Work out the finished part from the listing and answer in its coordinate system (mm). Face numbers are marked on the shaded views. A direction names the side the tool comes from. Give positions to 0.01 mm unless a question says otherwise; leave off trailing zeros. Loops run counter-clockwise (first coordinate to the right, second up) from the corner with the lowest first, then second, coordinate; pieces in that order, holes last.
from build123d import *

# Parameters (mm, degrees)
PAD033_DEPTH                = 10
PAD032_DEPTH                = 10
BOX026_W                    = 12
BOX026_H                    = 10
BOX026_DEPTH                = 30
CYLINDER036_R               = 2.2
CYLINDER036_DEPTH           = 18
CYLINDER036_ROLL_ANGLE      = -90
ARRAY006_X_COUNT            = 2
ARRAY006_X_PITCH            = 49.2
ARRAY006_Z_COUNT            = 2
ARRAY006_Z_PITCH            = 10.3
PAD021_DEPTH                = 6
PAD020_DEPTH                = 10
BOX027_W                    = 12
BOX027_H                    = 10
BOX027_DEPTH                = 30
CYLINDER037_R               = 2.2
CYLINDER037_DEPTH           = 18
CYLINDER037_ROLL_ANGLE      = -90
ARRAY007_X_COUNT            = 2
ARRAY007_X_PITCH            = 49.2
ARRAY007_Z_COUNT            = 2
ARRAY007_Z_PITCH            = 10.3
PAD023_DEPTH                = 6
PAD022_DEPTH                = 10
BOX025_W                    = 16.3
BOX025_H                    = 10
BOX025_DEPTH                = 17
SKETCH018_R                 = 3
PAD018_DEPTH                = 4
SKETCH019_R                 = 3
PAD019_DEPTH                = 4
BOX024_W                    = 20
BOX024_H                    = 17
BOX024_DEPTH                = 10
FILLET007_R                 = 1
FILLET007_ROLL_ANGLE        = 90
FILLET008_1_R               = 2
FILLET008_2_R               = 1
BOX018_W                    = 16.3
BOX018_H                    = 10
BOX018_DEPTH                = 17
SKETCH010_R                 = 3
PAD010_DEPTH                = 4
SKETCH011_R                 = 3
PAD011_DEPTH                = 4
BOX016_W                    = 20
BOX016_H                    = 17
BOX016_DEPTH                = 10
FILLET005_R                 = 1
FILLET005_ROLL_ANGLE        = 90
FILLET006_1_R               = 2
FILLET006_2_R               = 1
PAD009_DEPTH                = 26.3
FUSION009003041_PITCH_ANGLE = 90


with BuildPart() as obj1:
    # Sketch033 → Pad033 (new body)
    with BuildSketch(Plane(origin=(-28, -127, 4), x_dir=(1, 0, 0), z_dir=(0, 0, 1))):
        Polygon((0, 0), (0, 6), (26, 6), (26, 0), (23, 0), (23, 3), (3, 3), (3, 0), align=None)
    extrude(amount=PAD033_DEPTH)


with BuildPart() as obj1_mirror:
    # Part__Mirroring009: instance of obj1
    add(obj1.part.mirror(Plane(origin=(0, 0, 0), x_dir=(1, 0, 0), z_dir=(0, 1, 0))))


with BuildPart() as obj1_mirror_1:
    # Part__Mirroring009 placement: moved
    add(obj1_mirror.part.moved(Location((0, -130, 0))))


with BuildPart() as obj2:
    # Sketch032 → Pad032 (new body)
    with BuildSketch(Plane(origin=(-28, -127, 4), x_dir=(1, 0, 0), z_dir=(0, 0, 1))):
        Polygon((0, 0), (0, 6), (26, 6), (26, 0), (23, 0), (23, 3), (3, 3), (3, 0), align=None)
    extrude(amount=PAD032_DEPTH)

    # Fusion009003040: union obj1_mirror
    add(obj1_mirror_1.part)


with BuildPart() as obj3:
    # Box026 → Box026 (new body)
    with BuildSketch(Plane(origin=(-29.5, -13, 0), x_dir=(1, 0, 0), z_dir=(0, 0, 1))):
        with Locations((6, 5)):
            Rectangle(BOX026_W, BOX026_H)
    extrude(amount=BOX026_DEPTH)


with BuildPart() as obj4:
    # Cylinder036 → Cylinder036 (new body)
    with BuildSketch(Plane.XY):
        Circle(CYLINDER036_R)
    extrude(amount=CYLINDER036_DEPTH)


with BuildPart() as obj4_1:
    # Cylinder036 roll: moved
    add(obj4.part.rotate(Axis((0, 0, 0), (1, 0, 0)), CYLINDER036_ROLL_ANGLE))


with BuildPart() as obj4_2:
    # Cylinder036 placement: moved
    add(obj4_1.part.moved(Location((150.075, 41, 13.5))))

    # Array006 X: obj4_2


with BuildPart() as obj4_3:
    add(obj4_2.part)
    with Locations(*[(i * ARRAY006_X_PITCH, 0, 0) for i in range(1, ARRAY006_X_COUNT)]):
        add(obj4_2.part)

    # Array006 Z: obj4_2


with BuildPart() as obj4_4:
    add(obj4_3.part)
    with Locations(*[(0, 0, -i * ARRAY006_Z_PITCH) for i in range(1, ARRAY006_Z_COUNT)]):
        add(obj4_3.part)


with BuildPart() as obj5:
    # Sketch021 → Pad021 (new body)
    with BuildSketch(Plane(origin=(10, 54.8, 0), x_dir=(1, 0, 0), z_dir=(0, -1, 0))):
        Polygon((0, 18.5), (0, 24.5), (50.5, 24.5), (50.5, 0), (40.5, 0), (40.5, 18.5), align=None)
    extrude(amount=PAD021_DEPTH)


with BuildPart() as obj6:
    # Sketch020 → Pad020 (new body)
    with BuildSketch(Plane.YZ):
        Polygon((14, 0), (0, 0), (0, 24.5), (54.8, 24.5), (54.8, 0), (48.8, 0), (48.8, 18.5), (14, 18.5), align=None)
    extrude(amount=PAD020_DEPTH)

    # Fusion009003025: union obj5
    add(obj5.part)


with BuildPart() as obj6_1:
    # Fusion009003025 placement: moved
    add(obj6.part.moved(Location((144.425, -3, 0))))

    # Cut017: cut obj4
    add(obj4_4.part, mode=Mode.SUBTRACT)


with BuildPart() as obj6_2:
    # Cut017 placement: moved
    add(obj6_1.part.moved(Location((-172.725, -4, 0))))

    # Cut018: cut obj3
    add(obj3.part, mode=Mode.SUBTRACT)


with BuildPart() as obj7:
    # Box027 → Box027 (new body)
    with BuildSketch(Plane(origin=(-29.5, -13, 0), x_dir=(1, 0, 0), z_dir=(0, 0, 1))):
        with Locations((6, 5)):
            Rectangle(BOX027_W, BOX027_H)
    extrude(amount=BOX027_DEPTH)


with BuildPart() as obj8:
    # Cylinder037 → Cylinder037 (new body)
    with BuildSketch(Plane.XY):
        Circle(CYLINDER037_R)
    extrude(amount=CYLINDER037_DEPTH)


with BuildPart() as obj8_1:
    # Cylinder037 roll: moved
    add(obj8.part.rotate(Axis((0, 0, 0), (1, 0, 0)), CYLINDER037_ROLL_ANGLE))


with BuildPart() as obj8_2:
    # Cylinder037 placement: moved
    add(obj8_1.part.moved(Location((150.075, 41, 13.5))))

    # Array007 X: obj8_2


with BuildPart() as obj8_3:
    add(obj8_2.part)
    with Locations(*[(i * ARRAY007_X_PITCH, 0, 0) for i in range(1, ARRAY007_X_COUNT)]):
        add(obj8_2.part)

    # Array007 Z: obj8_2


with BuildPart() as obj8_4:
    add(obj8_3.part)
    with Locations(*[(0, 0, -i * ARRAY007_Z_PITCH) for i in range(1, ARRAY007_Z_COUNT)]):
        add(obj8_3.part)


with BuildPart() as obj9:
    # Sketch023 → Pad023 (new body)
    with BuildSketch(Plane(origin=(10, 54.8, 0), x_dir=(1, 0, 0), z_dir=(0, -1, 0))):
        Polygon((0, 18.5), (0, 24.5), (50.5, 24.5), (50.5, 0), (40.5, 0), (40.5, 18.5), align=None)
    extrude(amount=PAD023_DEPTH)


with BuildPart() as obj10:
    # Sketch022 → Pad022 (new body)
    with BuildSketch(Plane.YZ):
        Polygon((14, 0), (0, 0), (0, 24.5), (54.8, 24.5), (54.8, 0), (48.8, 0), (48.8, 18.5), (14, 18.5), align=None)
    extrude(amount=PAD022_DEPTH)

    # Fusion009003026: union obj9
    add(obj9.part)


with BuildPart() as obj10_1:
    # Fusion009003026 placement: moved
    add(obj10.part.moved(Location((144.425, -3, 0))))

    # Cut019: cut obj8
    add(obj8_4.part, mode=Mode.SUBTRACT)


with BuildPart() as obj10_2:
    # Cut019 placement: moved
    add(obj10_1.part.moved(Location((-172.725, -4, 0))))

    # Cut020: cut obj7
    add(obj7.part, mode=Mode.SUBTRACT)


with BuildPart() as obj11:
    # Part__Mirroring: instance of obj10
    add(obj10_2.part.mirror(Plane(origin=(0, 0, 0), x_dir=(1, 0, 0), z_dir=(0, 1, 0))))


with BuildPart() as obj11_1:
    # Part__Mirroring placement: moved
    add(obj11.part.moved(Location((0, -130, 0))))


with BuildPart() as obj12:
    # Box025 → Box025 (new body)
    with BuildSketch(Plane(origin=(-26.3, -8, 0), x_dir=(1, 0, 0), z_dir=(0, 0, 1))):
        with Locations((8.15, 5)):
            Rectangle(BOX025_W, BOX025_H)
    extrude(amount=BOX025_DEPTH)


with BuildPart() as obj13:
    # Sketch018 → Pad018 (new body)
    with BuildSketch(Plane.XY):
        with BuildLine():
            Line((0, 17), (20, 17))
            ThreePointArc((20, 0), (28.500019, 8.5), (20, 17))
            Line((20, 0), (0, 0))
            Line((0, 0), (0, 17))
        make_face()
        with Locations((20.000019, 8.5)):
            Circle(SKETCH018_R, mode=Mode.SUBTRACT)
    extrude(amount=PAD018_DEPTH)


with BuildPart() as obj14:
    # Sketch019 → Pad019 (new body)
    with BuildSketch(Plane.XY.offset(14)):
        with BuildLine():
            Line((0, 17), (20, 17))
            ThreePointArc((20, 0), (28.500019, 8.5), (20, 17))
            Line((20, 0), (0, 0))
            Line((0, 0), (0, 17))
        make_face()
        with Locations((20.000019, 8.5)):
            Circle(SKETCH019_R, mode=Mode.SUBTRACT)
    extrude(amount=PAD019_DEPTH)


with BuildPart() as obj15:
    # Box024 → Box024 (new body)
    with BuildSketch(Plane(origin=(-16, 0, 4), x_dir=(1, 0, 0), z_dir=(0, 0, 1))):
        with Locations((10, 8.5)):
            Rectangle(BOX024_W, BOX024_H)
    extrude(amount=BOX024_DEPTH)

    # Fusion009003021: union obj13, obj14
    add(obj13.part)
    add(obj14.part)

    # Fillet007
    fillet007_edges = [obj15.edges().sort_by_distance(p)[0] for p in [
        (0, 8.5, 18),
        (-16, 0, 9),
        (-16, 17, 9),
        (0, 8.5, 0),
    ]]
    fillet(fillet007_edges, radius=FILLET007_R)


with BuildPart() as obj15_1:
    # Fillet007 roll: moved
    add(obj15.part.rotate(Axis((0, 0, 0), (1, 0, 0)), FILLET007_ROLL_ANGLE))


with BuildPart() as obj15_2:
    # Fillet007 placement: moved
    add(obj15_1.part.moved(Location((16, 15, 0))))

    # Fillet008 1
    fillet008_1_edges = [obj15_2.edges().sort_by_distance(p)[0] for p in [
        (16, 1, 8.5),
        (16, 11, 8.5),
    ]]
    fillet(fillet008_1_edges, radius=FILLET008_1_R)

    # Fillet008 2
    fillet008_2_edges = [obj15_2.edges().sort_by_distance(p)[0] for p in [
        (20, 1, 8.5),
        (20, 11, 8.5),
    ]]
    fillet(fillet008_2_edges, radius=FILLET008_2_R)


with BuildPart() as obj15_3:
    # Fillet008 placement: moved
    add(obj15_2.part.moved(Location((-20, -9, 0))))

    # Fusion009003022: union obj12
    add(obj12.part)


with BuildPart() as obj15_4:
    # Fusion009003022 placement: moved
    add(obj15_3.part.moved(Location((0, -134, 0))))


with BuildPart() as obj16:
    # Box018 → Box018 (new body)
    with BuildSketch(Plane(origin=(-26.3, -8, 0), x_dir=(1, 0, 0), z_dir=(0, 0, 1))):
        with Locations((8.15, 5)):
            Rectangle(BOX018_W, BOX018_H)
    extrude(amount=BOX018_DEPTH)


with BuildPart() as obj17:
    # Sketch010 → Pad010 (new body)
    with BuildSketch(Plane.XY):
        with BuildLine():
            Line((0, 17), (20, 17))
            ThreePointArc((20, 0), (28.500019, 8.5), (20, 17))
            Line((20, 0), (0, 0))
            Line((0, 0), (0, 17))
        make_face()
        with Locations((20.000019, 8.5)):
            Circle(SKETCH010_R, mode=Mode.SUBTRACT)
    extrude(amount=PAD010_DEPTH)


with BuildPart() as obj18:
    # Sketch011 → Pad011 (new body)
    with BuildSketch(Plane.XY.offset(14)):
        with BuildLine():
            Line((0, 17), (20, 17))
            ThreePointArc((20, 0), (28.500019, 8.5), (20, 17))
            Line((20, 0), (0, 0))
            Line((0, 0), (0, 17))
        make_face()
        with Locations((20.000019, 8.5)):
            Circle(SKETCH011_R, mode=Mode.SUBTRACT)
    extrude(amount=PAD011_DEPTH)


with BuildPart() as obj19:
    # Box016 → Box016 (new body)
    with BuildSketch(Plane(origin=(-16, 0, 4), x_dir=(1, 0, 0), z_dir=(0, 0, 1))):
        with Locations((10, 8.5)):
            Rectangle(BOX016_W, BOX016_H)
    extrude(amount=BOX016_DEPTH)

    # Fusion009003009: union obj17, obj18
    add(obj17.part)
    add(obj18.part)

    # Fillet005
    fillet005_edges = [obj19.edges().sort_by_distance(p)[0] for p in [
        (0, 8.5, 18),
        (-16, 0, 9),
        (-16, 17, 9),
        (0, 8.5, 0),
    ]]
    fillet(fillet005_edges, radius=FILLET005_R)


with BuildPart() as obj19_1:
    # Fillet005 roll: moved
    add(obj19.part.rotate(Axis((0, 0, 0), (1, 0, 0)), FILLET005_ROLL_ANGLE))


with BuildPart() as obj19_2:
    # Fillet005 placement: moved
    add(obj19_1.part.moved(Location((16, 15, 0))))

    # Fillet006 1
    fillet006_1_edges = [obj19_2.edges().sort_by_distance(p)[0] for p in [
        (16, 1, 8.5),
        (16, 11, 8.5),
    ]]
    fillet(fillet006_1_edges, radius=FILLET006_1_R)

    # Fillet006 2
    fillet006_2_edges = [obj19_2.edges().sort_by_distance(p)[0] for p in [
        (20, 1, 8.5),
        (20, 11, 8.5),
    ]]
    fillet(fillet006_2_edges, radius=FILLET006_2_R)


with BuildPart() as obj19_3:
    # Fillet006 placement: moved
    add(obj19_2.part.moved(Location((-20, -9, 0))))

    # Fusion009003020: union obj16
    add(obj16.part)

    # Fusion009003023: union obj15
    add(obj15_4.part)


with BuildPart() as obj20:
    # Sketch009 → Pad009 (new body)
    with BuildSketch(Plane(origin=(0, 0, 0), x_dir=(0, 1, 0), z_dir=(-1, 0, 0))):
        with BuildLine():
            Line((-140, 0), (-140, 50))
            ThreePointArc((-120, 70), (-134.142136, 64.142136), (-140, 50))
            Line((-120, 70), (-20, 70))
            ThreePointArc((0, 50), (-5.857864, 64.142136), (-20, 70))
            Line((0, 50), (0, 0))
            Line((0, 0), (-8, 0))
            Line((-8, 0), (-8, 50))
            ThreePointArc((-8, 50), (-11.514719, 58.485281), (-20, 62))
            Line((-20, 62), (-120, 62))
            ThreePointArc((-120, 62), (-128.485281, 58.485281), (-132, 50))
            Line((-132, 50), (-132, 0))
            Line((-132, 0), (-140, 0))
        make_face()
    extrude(amount=PAD009_DEPTH)

    # Fusion009003024: union obj19
    add(obj19_3.part)


with BuildPart() as obj20_1:
    # Fusion009003024 placement: moved
    add(obj20.part.moved(Location((-2, 5, 0))))

    # Fusion009003027: union obj6, obj11
    add(obj6_2.part)
    add(obj11_1.part)

    # Fusion009003041: union obj2
    add(obj2.part)


with BuildPart() as obj20_2:
    # Fusion009003041 pitch: moved
    add(obj20_1.part.rotate(Axis((0, 0, 0), (0, 1, 0)), FUSION009003041_PITCH_ANGLE))


with BuildPart() as obj20_3:
    # Fusion009003041 placement: moved
    add(obj20_2.part.moved(Location((359, 67, 326))))


solid = obj20_3.part
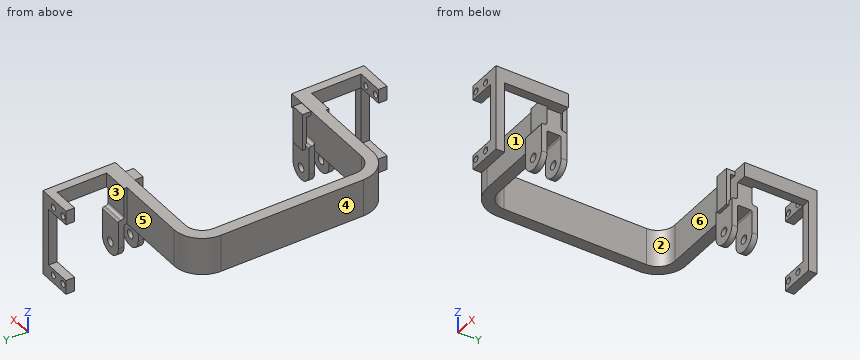
Item 1: Find section A-A, the plane x = 300. Write down the section's boundary in (y, z), plus the area to 3 significant figures.
Item 2: Find section D-D, the plane y = 30.5. Write down the section's boundary in (x, z).
Item 3: Consider line 1 (Y direction, x = 368, z = 309); line 2 (X direction, y = -107, z = 299); line 3 (Z direction, x = 367.5, y = -57.45). Determine where each line is inside the solid, lowest interval first.
Item 4: For the marked faces 1, 2 and 3, determine the directions among +Z, -Z, +X, -X, +Y, -Y from which every point of the face is accessible in a straight line to the end or side of a thin tool.
Item 5: Determine the mould class of the marked faces 4, 5 and 6 for opening direction X: released by +X, released by -X, zero draft, split by the parting line, or undercut.
Item 6: Flat-ended cylindrical pins translate along their axes: pin 1 Ø1.1 at (x, y) = (370.5, -57.5) entering from +Z; pin 2 Ø5 at (x, z) = (367.5, 337) entering from -Y; pin 3 Ø3 at (y, z) = (-108.5, 351.5) entering from -X; pin 4 Ø5 at (x, z) = (372.5, 348.65) entering from -Y. Find the tip coordinate at first contact, or state that the pin passes through.
Item 7: Find section B-B, the plane x = 367.5. Give the number of separate pieces and of enclosed holes in the cut face, plus the area to 3 significant figures.
Ans:
1. outline: (-65.86, 328) - (-55.94, 328) - (-55.94, 354.3) - (-65.86, 354.3) - close; (59.94, 328) - (69.86, 328) - (69.86, 354.3) - (59.94, 354.3) - close
1. area: 522 mm2
2. outline: (289, 328) - (297, 328) - (297, 354.3) - (289, 354.3) - close
3. line 1: y = -74 to -70, -60 to -56, 60 to 64, 74 to 78
3. line 2: x = 359 to 360.05, 364.35 to 370.35, 374.65 to 383.5
3. line 3: z = 303.5 to 309, 315 to 332, 351 to 354
4. face 1: +Z, -Z, -X, -Y
4. face 2: +Z, -Z
4. face 3: +Z, -X
5. face 4: released by -X
5. face 5: zero draft
5. face 6: undercut
6. pin 1: stops at z = 354
6. pin 2: stops at y = -70
6. pin 3: stops at x = 359
6. pin 4: stops at y = -110.8
7. separate pieces: 10
7. enclosed holes: 2
7. area: 1,300 mm2
